The listing builds one solid part. Answer for the finished solid, in the listing's coordinates (mm). A direction names the side the tool comes from. Give positions to 0.01 mm unless a question says otherwise; leave off trailing zeros. Loops run counter-clockwise (first coordinate to the right, second up) from the corner with the lowest first, then second, coordinate; pieces in that order, holes last.
Item 1: Section B-B, the plane x = -2.5 is taken. Give the vertices of the cut face in (y, z).
Item 2: Consider line 1 along Z through (x, y) = (19, 5.5); line 2 along X through (y, z) = (5.5, -30); line 3 along X through (y, z) = (22, 32). Determine where each line is inside the solid, lowest interval first.
Item 3: Section C-C, the plane z = -3.5 is taken. Give the vertices of the cut face in (x, y).
Item 4: Each of these flat-tipped pins is pushed along its axis until it touches: pin 1 Ø10 at (x, y) = (2.5, 20) entering from +Z; pin 2 Ø6 at (x, y) = (12, 13.5) entering from -Z; pin 3 Ø10 at (y, z) = (16.5, 4) entering from -X. Where does it stop, or does it pass through?
Item 5: A tool of negligible diameter and unlimited length cuts with its end or side. For faces 5 (the face through (0, 5, 0)), 6 (the face through (-25, 6, -25)), 7 (the face through (0, 6, 1.5)), 8 (the face through (26, 19, -25)), from which of +Z, -Z, +X, -X, +Y, -Y can it reach the whole face along a straight path? Write none if from no direction.
Item 6: Section A-A, the plane y = 10.5 is taken. Give the vertices of the cut face in (x, z).
Item 7: The mould has two halves that part along Y. Classify faces 1 (the face through (0, 6, -0.5)), 2 (the face through (25, 6, 27)), 3 (the face through (0, 0, -1)), 4 (the face through (-30, 2, 1)): pulls with the +Y half, pulls with the -Y half, needs draft (parallel to the pull), parting line crosses it, or undercut.
from build123d import *

# Parameters (mm, degrees)
SKETCH1_W           = 60
SKETCH1_H           = 113
BOSS_EXTRUDE1_DEPTH = 5
SKETCH2_W           = 50
SKETCH2_H           = 50
BOSS_EXTRUDE3_DEPTH = 2
LPATTERN1_COUNT     = 2
LPATTERN1_PITCH     = 52
SKETCH3_W           = 52
SKETCH3_H           = 51.9
BOSS_EXTRUDE8_DEPTH = 25
LPATTERN5_COUNT     = 2
LPATTERN5_PITCH     = 52


with BuildPart() as part:
    # Sketch1 → Boss-Extrude1 (new body)
    with BuildSketch(Plane(origin=(0, 0, 0), x_dir=(1, 0, 0), z_dir=(0, 1, 0))):
        Rectangle(SKETCH1_W, SKETCH1_H)
    extrude(amount=BOSS_EXTRUDE1_DEPTH)

    # Sketch2 → Boss-Extrude3 (add)
    with BuildSketch(Plane(origin=(0, 5, 0), x_dir=(1, 0, 0), z_dir=(0, 1, 0))):
        with Locations((0, -26.5)):
            Rectangle(SKETCH2_W, SKETCH2_H)
    boss_extrude3 = extrude(amount=BOSS_EXTRUDE3_DEPTH)

    # LPattern1: Boss-Extrude3 ×2
    with Locations(*[(0, 0, -i * LPATTERN1_PITCH) for i in range(1, LPATTERN1_COUNT)]):
        add(boss_extrude3)

    # Sketch3 → Boss-Extrude8 (add)
    with BuildSketch(Plane(origin=(0, 7, 0), x_dir=(1, 0, 0), z_dir=(0, 1, 0))):
        with Locations((0, -26.55)):
            Rectangle(SKETCH3_W, SKETCH3_H)
    boss_extrude8 = extrude(amount=BOSS_EXTRUDE8_DEPTH)

    # LPattern5: Boss-Extrude8 ×2
    with Locations(*[(0, 0, -i * LPATTERN5_PITCH) for i in range(1, LPATTERN5_COUNT)]):
        add(boss_extrude8)


solid = part.part
Worked answers:
1. outline: (0, -56.5) - (5, -56.5) - (5, -50.5) - (7, -50.5) - (7, -51.4) - (32, -51.4) - (32, 0.5) - (7, 0.5) - (7, -0.5) - (5, -0.5) - (5, 1.5) - (7, 1.5) - (7, 0.6) - (32, 0.6) - (32, 52.5) - (7, 52.5) - (7, 51.5) - (5, 51.5) - (5, 56.5) - (0, 56.5) - close
2. line 1: z = -50.5 to -0.5, 1.5 to 51.5
2. line 2: x = -25 to 25
2. line 3: x = -26 to 26
3. outline: (-30, 0) - (30, 0) - (30, 5) - (25, 5) - (25, 7) - (26, 7) - (26, 32) - (-26, 32) - (-26, 7) - (-25, 7) - (-25, 5) - (-30, 5) - close
4. pin 1: stops at z = 52.5
4. pin 2: stops at z = -51.4
4. pin 3: stops at x = -26
5. face 5: none
5. face 6: +Z, -Z, -X
5. face 7: +X, -X
5. face 8: +Z, -Z, +X, +Y
6. outline: (-26, -51.4) - (26, -51.4) - (26, 0.5) - (-26, 0.5) - close; (-26, 0.6) - (26, 0.6) - (26, 52.5) - (-26, 52.5) - close
7. face 1: undercut
7. face 2: undercut
7. face 3: pulls with the -Y half
7. face 4: needs draft
